Autodesk Inventor part; units mm, degrees
ref_plane "YZ Plane" through (0, 0, 0) normal (1, 0, 0) x (0, 1, 0)
ref_plane "XZ Plane" through (0, 0, 0) normal (0, 1, 0) x (-1, 0, 0)
ref_plane "XY Plane" through (0, 0, 0) normal (0, 0, 1) x (1, 0, 0)
sketch "Sketch1" plane through (0, 0, 0) normal (0, 0, 1) x (1, 0, 0)
  line L0 (-50, -61.1941) -> (50, -61.1941)
  line L1 (50, -61.1941) -> (50, 61.1941)
  line L2 (50, 61.1941) -> (-50, 61.1941)
  line L3 (-50, 61.1941) -> (-50, -61.1941)
  line L4 (-50, -61.1941) -> (50, 61.1941) construction
  line L5 (50, -61.1941) -> (-50, 61.1941) construction
  point P0 (0, 0)
  dimension "d0" = 100
  dimension "d1" = 122.3883
extrude "Plate1" add sketch "Sketch1" along normal blind 6
fillet "Corner Round1" radius 20 4 edges at (50, -61.1941, 3) (-50, -61.1941, 3) (-50, 61.1941, 3) (50, 61.1941, 3)
sketch "Sketch5" plane through (0, 0, 6) normal (0, 0, 1) x (1, 0, 0)
  line L0 (50, 41.1941) -> (50, -41.1941)
  line L1 (50, 31.1941) -> (-50, 31.1941)
  line L2 (-50, -41.1941) -> (-50, 41.1941)
  line L3 (-30, 61.1941) -> (30, 61.1941)
  point P0 (0, 0)
  dimension "d23" = 30
feature "Fold1" [suppressed]
equation "\"d1\" = Legs_Upper_plate_lenght"
equation "\"d2\" = Thickness"
equation "\"d24\" = BendReliefWidth"
equation "\"d25\" = BendReliefDepth"
equation "\"d26\" = MinimumRemnant"
equation "\"d27\" = TransitionRadius"
equation "\"d29\" = BendRadius"
equation "\"BendReliefWidth\" = Thickness"
equation "\"BendReliefDepth\" = 0.5 * Thickness"
equation "\"CornerReliefSize\" = 4 * Thickness"
equation "\"MinimumRemnant\" = 2 * Thickness"
equation "\"TransitionRadius\" = BendRadius"
equation "\"JacobiRadiusSize\" = BendRadius"
equation "\"GapSize\" = Thickness"
properties part number "PRS 9694 leg plate for filter_D1200" material "Stainless Steel"
Part model, mm, in its own coordinate system. Round coordinates to 2 decimals unless told otherwise and drop trailing zeros. Loops run counter-clockwise (first coordinate to the right, second up) from the corner with the lowest first, then second, coordinate; pieces in that order, holes last. Notation, with made-up numbers: (8, 35) -> (32, 35) arc R30 ccw to (32, 62) -> close; hole circle Ø11 at (80.25, 17). An arc over 180 degrees is marked (long way). Use CSV: the item, a comma, the result in double quotes. Start each with the question number.
1) Wall check: L1, parallel to X at y = -42, z = 3.85; L2, parallel to X at y = 44, z = 3.55; L3, parallel to Y at x = 34, z = 3.65. Give the ranges that are in metal, low to high. Write a range as [from, to].
2) Cut at B-B, the plane x = 39.5. Write the cut outline in (y, z), plus the area to 3 significant figures.
3) Cut at A-A, the plane z = 2.7. Write the cut outline in (x, y).
4) Cut at C-C, the plane y = -52. Write the cut outline in (x, z), plus the area to 3 significant figures.
Determined:
1,L1,"x = [-49.98, 49.98]"
1,L2,"x = [-49.8, 49.8]"
1,L3,"y = [-60.79, 60.79]"
2,outline,"(-58.79, 0) -> (58.79, 0) -> (58.79, 6) -> (-58.79, 6) -> close"
2,area,"706 mm2"
3,outline,"(-50, -41.19) arc R20 ccw to (-30, -61.19) -> (30, -61.19) arc R20 ccw to (50, -41.19) -> (50, 41.19) arc R20 ccw to (30, 61.19) -> (-30, 61.19) arc R20 ccw to (-50, 41.19) -> close"
4,outline,"(-46.83, 0) -> (46.83, 0) -> (46.83, 6) -> (-46.83, 6) -> close"
4,area,"562 mm2"
